The model under review builds one solid part; all positions refer to its coordinate system, in mm. Coordinates: 2 decimals unless noted, no trailing zeros. Write each loop counter-clockwise with the first axis right and the second up, starting at its lowest first coordinate (ties: lowest second). Pieces come first, ordered by that corner, then holes. Notation, with made-up numbers: (23.25, 25) - (44.25, 25) arc R30 cw to (44.25, 47) - close; hole circle Ø8 at (11.5, -33.75). An arc over 180 degrees is marked (long way). Use one line per item in the form item = value. Start each with the question number.
```python
from build123d import *

# Parameters (mm, degrees)
F1_DEPTH = 20
F3_DEPTH = 100
F4_R     = 5


with BuildPart() as f1:
    # F0 (on Front) → F1 (new body)
    with BuildSketch(Plane.XZ):
        with BuildLine():
            Line((91.030714, 28.54419), (-98.969286, 28.54419))
            Line((-98.969286, 28.54419), (-98.969286, -70.923594))
            ThreePointArc((-98.969286, -70.923594), (-4.0099, -85.688886), (91.030714, -71.45581))
            Line((91.030714, -71.45581), (91.030714, 28.54419))
        make_face()
    extrude(amount=F1_DEPTH)

    # F2 (on Right) → F3 (cut, symmetric)
    with BuildSketch(Plane.YZ):
        with BuildLine():
            ThreePointArc((0, -41.784719), (-0.601025, -60.211753), (-15.13516, -71.555287))
            Line((-15.13516, -71.555287), (-19.817429, -85.876599))
            Line((-19.817429, -85.876599), (3.398273, -87.581709))
            Line((3.398273, -87.581709), (10.874517, -61.349276))
            Line((10.874517, -61.349276), (0, -41.784719))
        make_face()
    extrude(amount=F3_DEPTH, both=True, mode=Mode.SUBTRACT)

    # F4
    f4_edges = [f1.edges().sort_by_distance(p)[0] for p in [
        (91.030714, -10, 28.54419),
        (-3.969286, 0, 28.54419),
        (-98.969286, 0, -15.191684),
        (-98.969286, -10, 28.54419),
        (91.030714, 0, -15.191684),
    ]]
    fillet(f4_edges, radius=F4_R)


solid = f1.part
```
1. For L1, parallel to Z at x = -28.5, y = -12.5; L2, parallel to Z at x = 28, y = -2.25; L3, parallel to X at y = -2.5, z = 22, list the stretches that pass through material, from the lowest coordinate up.
2. Take a section at A-A (x = 68). State the section outline as (y, z) points, plus the area to 3 significant figures.
3. For P1, Ø1, axis at x = -29.5, y = -13.5, coming from the -Z side; P2, Ø1.5, axis at x = -64.5, z = -69.5, coming from the +Y side; P3, Ø12, axis at x = 31.5, y = -14.5, coming from the -Z side, all flat-tipped, find the tip position at first contact; note any pin that passes through.
4. Take a section at B-B (y = -8). State the section outline as (x, z) points.
5. Take a section at C-C (x = -83.5). State the section outline as (y, z) points.
Returned:
q1.L1 = -70.77 to 28.54
q1.L2 = -62.94 to 27.72
q1.L3 = -98.3 to 90.36
q2.outline = (-20, -77.65) - (-17.13, -77.65) - (-15.14, -71.56) arc R21.75 ccw to (0, -58.93) - (0, 23.54) arc R5 ccw to (-5, 28.54) - (-20, 28.54) - close
q2.area = 1,960 mm²
q3.P1 = -71.26
q3.P2 = -8.38
q3.P3 = -84.18
q4.outline = (-98.97, -68.5) - (91.03, -68.5) - (91.03, 23.54) arc R5 ccw to (86.03, 28.54) - (-93.97, 28.54) arc R5 ccw to (-98.97, 23.54) - close
q5.outline = (-20, -75.38) - (-16.39, -75.38) - (-15.14, -71.56) arc R21.75 ccw to (0, -58.93) - (0, 23.54) arc R5 ccw to (-5, 28.54) - (-20, 28.54) - close
